Here's how the part is built. I have some questions about the finished solid (model axes, mm). A direction names the side the tool comes from. Round coordinates to 2 decimals unless told otherwise and drop trailing zeros. Write each loop counter-clockwise with the first axis right and the second up, starting at its lowest first coordinate (ties: lowest second). Pieces come first, ordered by that corner, then holes. Notation, with made-up numbers: (69, 82) -> (103, 82) arc R23 cw to (103, 117) -> close; hole circle Ø5 at (21.5, 88). An arc over 180 degrees is marked (long way). Answer as CSV lines item,"result".
```python
from build123d import *

# Parameters (mm, degrees)
F0_R     = 19.05
F0_R_2   = 9.525
F1_DEPTH = 1
F0_R_3   = 7.14375
F2_DEPTH = 0.25
F3_DEPTH = 1
F4_DEPTH = 0.75


with BuildPart() as f1:
    # F0 (on Top) → F1 (new body)
    with BuildSketch(Plane.XY):
        Circle(F0_R)
        Circle(F0_R_2, mode=Mode.SUBTRACT)
    extrude(amount=-F1_DEPTH)



with BuildPart() as f2:
    # F0 (on Top) → F2 (new body)
    with BuildSketch(Plane.XY):
        Circle(F0_R_2)
        Circle(F0_R_3, mode=Mode.SUBTRACT)
    extrude(amount=F2_DEPTH)

    # F0 (on Top) → F3 (join)
    with BuildSketch(Plane.XY):
        Circle(F0_R_3)
    extrude(amount=F3_DEPTH)


with BuildPart() as f1_1:
    add(f1.part)

    add(f2.part)  # F4 merges F2
    # F0 (on Top) → F4 (join)
    with BuildSketch(Plane.XY):
        Circle(F0_R_2)
        Circle(F0_R_3, mode=Mode.SUBTRACT)
    extrude(amount=-F4_DEPTH)


with BuildPart() as f5_1:
    # F5: copy of F1
    add(f1_1.part.moved(Location((0, 0, -6.35))))


solid = f1_1.part
```
1. For pin 1 Ø13 at (x, y) = (0, 0) entering from -Z; pin 2 Ø2 at (x, y) = (10.5, -4.5) entering from +Z, each with a flat end and sliding along its axis, tell me the tip position at first contact or that it passes through.
Numbers:
pin 1,"stops at z = 0"
pin 2,"stops at z = 0"
2. Suppose I cut it at A-A on x = 0. Please give me the cut outline in (y, z) (3 decimals), and give its area (3 significant figures).
Numbers:
outline,"(-19.05, -1) -> (-9.525, -1) -> (-9.525, -0.75) -> (-7.144, -0.75) -> (-7.144, 0) -> (7.144, 0) -> (7.144, -0.75) -> (9.525, -0.75) -> (9.525, -1) -> (19.05, -1) -> (19.05, 0) -> (9.525, 0) -> (9.525, 0.25) -> (7.144, 0.25) -> (7.144, 1) -> (-7.144, 1) -> (-7.144, 0.25) -> (-9.525, 0.25) -> (-9.525, 0) -> (-19.05, 0) -> close"
area,"38.1 mm^2"
3. Suppose I cut it at D-D on y = 14. Please give me the cut outline in (x, z).
Numbers:
outline,"(-12.92, -1) -> (12.92, -1) -> (12.92, 0) -> (-12.92, 0) -> close"
4. If we mould it in two halves opening along Y, with no side actions, what happens to faces 1 (the face through (4, 9, 0)), 2 (the face through (-15.12, -11.59, -0.49)), 3 (the face through (0, 0, 0))? For each: released by +Y, released by -Y, zero draft, split by the parting line, or undercut.
Numbers:
face 1,"zero draft"
face 2,"split by the parting line"
face 3,"undercut"
5. Suppose I cut it at C-C on z = -0.3. Please give me the cut outline in (x, y), and give its area (3 significant figures).
Numbers:
outline,"circle Ø38.1 at (0, 0); hole circle Ø14.29 at (0, 0)"
area,"980 mm^2"
6. If I drill on line 1 (Y direction, x = 0, z = -0.5); line 2 (Y direction, x = 0, z = -0.9) (3 decimals); line 3 (Z direction, x = -5, y = -9), over which ranges is the centre line in solid material (lowest first)?
Numbers:
line 1,"y = -19.05 to -7.14, 7.14 to 19.05"
line 2,"y = -19.05 to -9.525, 9.525 to 19.05"
line 3,"z = -1 to 0"
7. On a 3-axis mill with a long thin cutter (end or side, diameter ignored), from which of +Z, -Z, +X, -X, +Y, -Y can I reach the whole of each face in a straight line? I mean faces 4 (the face through (4, 9, -1)), 5 (the face through (3.5, 6.4, 0.25)), 6 (the face through (3.5, 6.4, -0.75)). Say none if no direction works.
Numbers:
face 4,"-Z, +X, -X, +Y, -Y"
face 5,"+Z"
face 6,"-Z"
